from build123d import *

# Parameters (mm, degrees)
SKETCH1_R               = 27
BOSS_EXTRUDE1_DEPTH     = 37.5
CUT_EXTRUDE2_DEPTH      = 54.518688325
CUT_EXTRUDE2_DEPTH_BACK = 54.518688325
SKETCH3_R               = 7.5
REVOLVE1_ANGLE          = 180
SKETCH2_R               = 22
CUT_EXTRUDE3_DEPTH      = 76
SKETCH13_R              = 1.5
BOSS_EXTRUDE3_DEPTH     = 5
CIRPATTERN1_COUNT       = 4


with BuildPart() as part:
    # Sketch1 → Boss-Extrude1 (new, symmetric)
    with BuildSketch(Plane.XY):
        Circle(SKETCH1_R)
    extrude(amount=BOSS_EXTRUDE1_DEPTH, both=True)

    # Sketch3 → Cut-Extrude2 (cut, two sides: drawn at the far end of the back side and taken through both)
    with BuildSketch(Plane(origin=(0, 0, 0), x_dir=(0, 0, -1), z_dir=(1, 0, 0)).offset(-CUT_EXTRUDE2_DEPTH_BACK)):
        with Locations((17.5, -3)):
            Circle(SKETCH3_R)
    extrude(amount=CUT_EXTRUDE2_DEPTH + CUT_EXTRUDE2_DEPTH_BACK, mode=Mode.SUBTRACT)

    # Sketch7 → Revolve1 (revolve)
    with BuildSketch(Plane(origin=(0, 0, -37.5), x_dir=(-1, 0, 0), z_dir=(0, 0, -1))):
        with BuildLine():
            Line((0, 27), (0, -27))
            ThreePointArc((0, -27), (-27, 0), (0, 27))
        make_face()
    revolve(axis=Axis((0, 27, -37.5), (0, 1, 0)), revolution_arc=REVOLVE1_ANGLE)

    # Sketch2 → Cut-Extrude3 (cut)
    with BuildSketch(Plane.XY.offset(37.5)):
        Circle(SKETCH2_R)
    extrude(amount=-CUT_EXTRUDE3_DEPTH, mode=Mode.SUBTRACT)

    # Sketch13 → Boss-Extrude3 (add)
    with BuildSketch(Plane.XY.offset(37.5)):
        with BuildLine():
            ThreePointArc((-21.444531116, 4.912441881), (-22, 0), (-21.444531116, -4.912441881))
            add(Edge.make_bspline(
                [(-21.444531116, -4.912441881), (-8.186572838, -4.722538036), (-8.186572838, 0), (-8.186572838, 4.722538036), (-21.444531116, 4.912441881)],
                knots=[1.611019415, 1.611019415, 1.611019415, 3.141592654, 3.141592654, 4.672165893, 4.672165893, 4.672165893], degree=2, weights=[1, 0.721183833, 1, 0.721183833, 1]))
        make_face()
        with Locations((-16, 0)):
            Circle(SKETCH13_R, mode=Mode.SUBTRACT)
    boss_extrude3 = extrude(amount=-BOSS_EXTRUDE3_DEPTH)

    # CirPattern1: Boss-Extrude3 ×4 about axis
    cirpattern1_axis = Axis((0, 0, 37.5), (0, 0, -1))
    for i in range(1, CIRPATTERN1_COUNT):
        add(boss_extrude3.rotate(cirpattern1_axis, i * 360 / CIRPATTERN1_COUNT))


solid = part.part
Build history of the part. All positions in model axes, mm. A direction names the side the tool comes from. Round coordinates to 2 decimals unless told otherwise and drop trailing zeros. Write each loop counter-clockwise with the first axis right and the second up, starting at its lowest first coordinate (ties: lowest second). Pieces come first, ordered by that corner, then holes. Notation, with made-up numbers: (-35, 76) - (-2, 76) arc R15 ccw to (-2, 101) - close; hole circle Ø3 at (-11, 23). An arc over 180 degrees is marked (long way). One line per question, with ' | ' between items.
1. Band-saw the part on A-A, the plane z = -17.5. Write the cut outline in (x, y), and give its area (3 significant figures).
Results are:
outline: (-26.62, 4.5) - (-21.53, 4.5) arc R22 cw to (21.53, 4.5) - (26.62, 4.5) arc R27 ccw to start; (-24.87, -10.5) arc R27 ccw to (24.87, -10.5) - (19.33, -10.5) arc R22 cw to (-19.33, -10.5) - close | area: 616 mm^2
2. Drop flat-ended pins along their axis: pin 1 Ø6 at (x, z) = (-18.5, 18) entering from -Y; pin 2 Ø6 at (x, z) = (7.5, -15) entering from -Y; pin 3 Ø3 at (x, y) = (0, -13) entering from -Z. Give the stop position or say it passes through.
Results are:
pin 1: y = -22.11 | pin 2: y = -26.62 | pin 3: z = -61.93
3. Drill centre lines: line 1 along X through (y, z) = (16, 34.1); line 2 along X through (y, z) = (20, 17.5). Where is each one in solid material? Low to high. Write a range as from..to.
Results are:
line 1: -21.75..-15.1, -4.43..-1.5, 1.5..4.43, 15.1..21.75 | line 2: -18.14..-9.17, 9.17..18.14
4. Tool access for faces 1 (the face through (0, 0, -38.5)), 2 (the face through (-0.07, -17.5, 35.03)), 3 (the face through (14.515, 22.767, 0.525)): list every direction of +Z, -Z, +X, -X, +Y, -Y with a clear straight run to the whole face (end or side of a thin tool).
Results are:
face 1: none | face 2: +Z | face 3: +Z, -Z
5. Band-saw the part on B-B, the plane x = 0. Give the number of separate pieces and of enclosed holes in the cut face, and give its area (3 significant figures).
Results are:
separate pieces: 3 | enclosed holes: 0 | area: 1,960 mm^2
6. Mould opens along Z. For faces 4 (the face through (20.984, 6.608, 0.032)), 5 (the face through (-12, 0, 37.5)), 6 (the face through (-18, 0, 32.5)), 7 (the face through (17.5, -0.07, 35.03)) say: released by +Z, released by -Z, zero draft, split by the parting line, or undercut.
Results are:
face 4: undercut | face 5: released by +Z | face 6: undercut | face 7: zero draft
